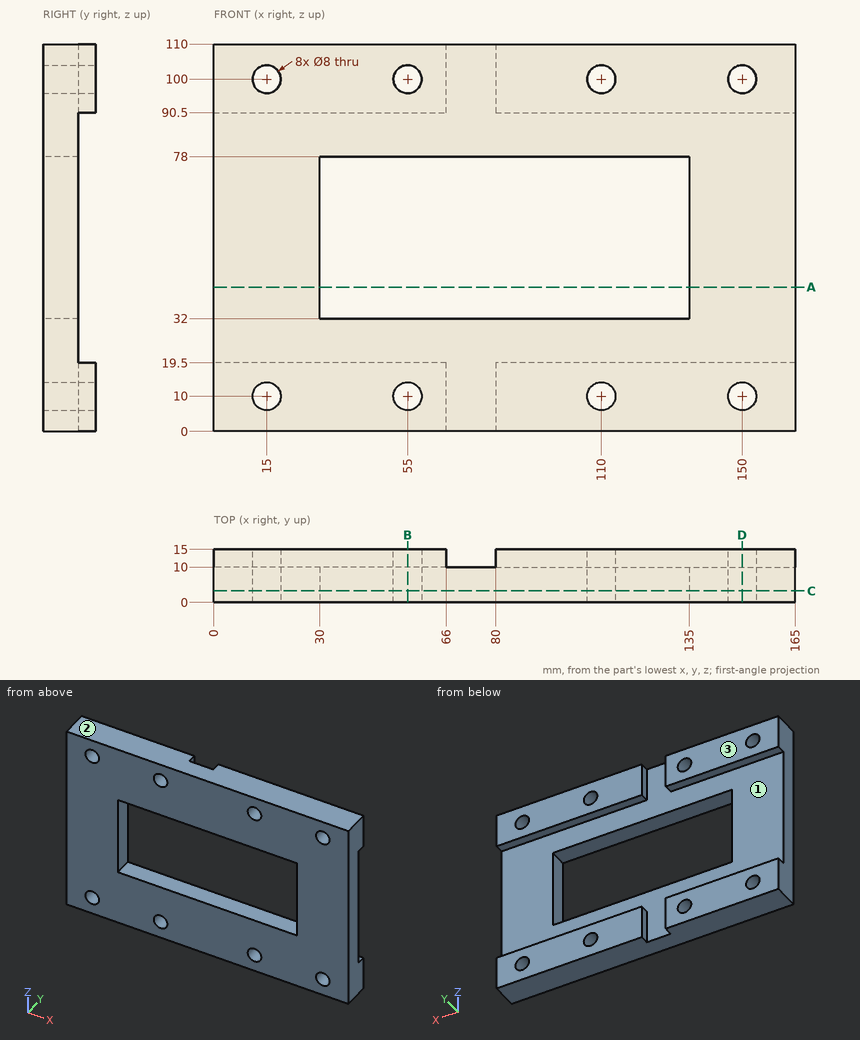
Input: dimensioned drawing with shaded views. Units: mm. Origin: part minimum x, y, z. Round coordinates to 2 decimals unless told otherwise and drop trailing zeros. Loops run counter-clockwise (first coordinate to the right, second up) from the corner with the lowest first, then second, coordinate; pieces in that order, holes last.
1) Pin query (flat end, axial travel): pin 1 (7 mm diameter, centred on x = 15, z = 100, fed in from +Y); pin 2 (5 mm diameter, centred on y = 6, z = 62, fed in from -X). Return the tip coordinate at first contact, or that it passes through.
Ans:
pin 1: passes through
pin 2: stops at x = 0
2) Section query C-C on y = 3.25. Count the separate pieces of the cut face and the enclosed holes in it, plus the area to 3 significant figures.
Ans:
separate pieces: 1
enclosed holes: 9
area: 12,900 mm2
3) Material intervals for line 1 (X direction, y = 4.25, z = 10); line 2 (Z direction, x = 110, y = 4.5); line 3 (X direction, y = 10.25, z = 100), sorted ascending.
Ans:
line 1: x = 0 to 11, 19 to 51, 59 to 106, 114 to 146, 154 to 165
line 2: z = 0 to 6, 14 to 32, 78 to 96, 104 to 110
line 3: x = 0 to 11, 19 to 51, 59 to 66, 80 to 106, 114 to 146, 154 to 165
4) Section query D-D on x = 150. Return the cut outline in (y, z), plus the area to 4 significant figures.
Ans:
outline: (0, 0) - (15, 0) - (15, 6) - (0, 6) - close; (0, 14) - (15, 14) - (15, 19.5) - (10, 19.5) - (10, 90.5) - (15, 90.5) - (15, 96) - (0, 96) - close; (0, 104) - (15, 104) - (15, 110) - (0, 110) - close
area: 1,055 mm2
5) Section query B-B on x = 55. Return the cut outline in (y, z), plus the area to 3 significant figures.
Ans:
outline: (0, 0) - (15, 0) - (15, 6) - (0, 6) - close; (0, 14) - (15, 14) - (15, 19.5) - (10, 19.5) - (10, 32) - (0, 32) - close; (0, 78) - (10, 78) - (10, 90.5) - (15, 90.5) - (15, 96) - (0, 96) - close; (0, 104) - (15, 104) - (15, 110) - (0, 110) - close
area: 595 mm2
6) Section query A-A on z = 41. Return the cut outline in (x, y).
Ans:
outline: (0, 0) - (30, 0) - (30, 10) - (0, 10) - close; (135, 0) - (165, 0) - (165, 10) - (135, 10) - close
7) Pull-direction query (Z, two-part tool) for the marked faces 1, 2 and 3; classes: released by +Z, released by -Z, zero draft, split by the parting line, or undercut.
Ans:
face 1: undercut
face 2: released by +Z
face 3: zero draft
